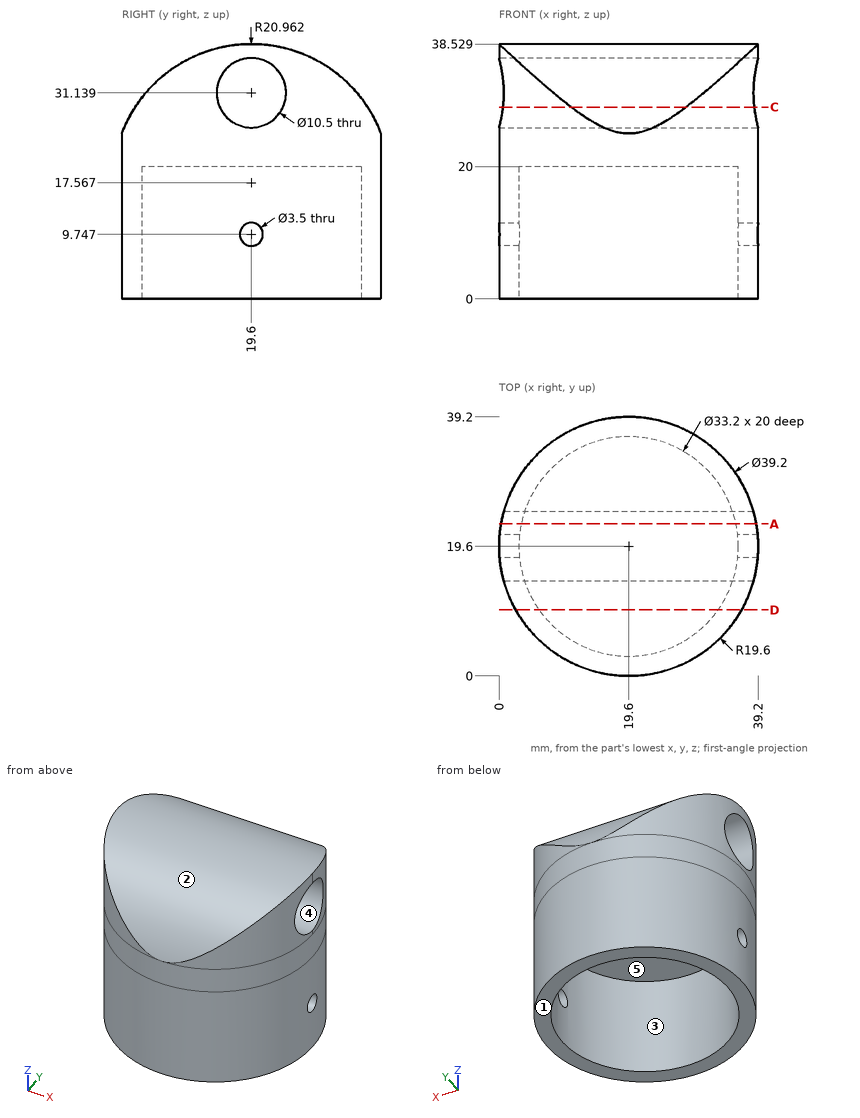
Source: three-view drawing plus pictorial views. Frame: mm from the lowest corner of the part. A direction names the side the tool comes from. Round coordinates to 2 decimals unless told otherwise and drop trailing zeros. Loops run counter-clockwise (first coordinate to the right, second up) from the corner with the lowest first, then second, coordinate; pieces in that order, holes last. Notation, with made-up numbers: M -1.5,53 L 15.5,53 A8 cw 15.5,58 Z; hole C 50,-23.5 d2. An arc over 180 degrees is marked long. Put each result on its own line as item: value.
(1) Pull-direction query (Y, two-part tool) for the marked faces 1, 2 and 3; classes: released by +Y, released by -Y, zero draft, split by the parting line, or undercut.
Solutions:
face 1: zero draft
face 2: split by the parting line
face 3: undercut
(2) Access query for the marked faces 4 and 5. Directions: +Z, -Z, +X, -X, +Y, -Y. A direction counts if a zero-diameter tool reaches every point of the face in a straight line with its end or side. Return the directions, or none.
Solutions:
face 4: +X, -X
face 5: -Z
(3) Ray query, line 1 (Z direction, x = 1, y = 19) (1 decimal); line 2 (X direction, y = 19, z = 12); line 3 (Y direction, x = 30, z = 23.5). Return the intervals inside material, ascending. Write a range as [from, to].
Solutions:
line 1: [0, 8.1], [11.4, 25.9], [36.4, 38.5]
line 2: [0.01, 3.01], [36.19, 39.19]
line 3: [2.99, 36.21]
(4) First-contact query: pin 1 (2 mm diameter, centred on x = 25, z = 9.5, fed in from -Y); pin 2 (5 mm diameter, centred on y = 16.5, z = 21.5, fed in from +X); pin 3 (12 mm diameter, centred on x = 6, y = 4.5, fed in from +Z). Flat tips, straight axial feed; report the tip coordinate or a pass-through.
Solutions:
pin 1: y = 0.5
pin 2: x = 39.19
pin 3: z = 36.45
(5) Section D-D, the plane y = 10. Return loops of the section in (x, z).
Solutions:
outline: M 2.51,0 L 6.06,0 L 6.06,20 L 33.14,20 L 33.14,0 L 36.69,0 L 36.69,36.2 L 2.51,36.2 Z
(6) Section C-C, the plane z = 29. Return loops of the section in (x, y) (1 decimal).
Solutions:
outline: M 0.6,14.8 A19.6 ccw 10.9,2 L 28.3,2 A19.6 ccw 38.6,14.8 Z; M 0.6,24.4 L 38.6,24.4 A19.6 ccw 28.3,37.2 L 10.9,37.2 A19.6 ccw Z
(7) Section A-A, the plane y = 23. Return loops of the section in (x, z), and give its area (3 significant figures).
Solutions:
outline: M 0.3,0 L 3.35,0 L 3.35,20 L 35.85,20 L 35.85,0 L 38.9,0 L 38.9,27.14 L 0.3,27.14 Z; M 0.3,35.14 L 38.9,35.14 L 38.9,38.25 L 0.3,38.25 Z
area: 518 mm²
